For this review, take the finished solid that the model builds, in its own axes (mm). A direction names the side the tool comes from. Give positions to 0.01 mm unless a question says otherwise; leave off trailing zeros. Loops run counter-clockwise (first coordinate to the right, second up) from the corner with the lowest first, then second, coordinate; pieces in that order, holes last. Notation, with made-up numbers: (-32, -26.75) - (25, -26.75) arc R23 ccw to (25, 6.25) - close; hole circle Ø4 at (36.25, 19.5). An arc over 180 degrees is marked (long way). Use CSV: the item, a comma, the result in double quotes. Start each with the question number.
1. Wall thickness on line 1 (Y direction, x = 0.5, z = -2.25); line 2 (Z direction, x = 2.5, y = 14.5); line 3 (Y direction, x = 1, z = -1): over which ranges is each line inside the solid? List them lowest first.
2. Mouldability with a two-part tool opening along X and no side actions: class faces 1 (the cylindrical face through (0.41, 6.26, 1.86)), 2 (the flat face through (-1.25, 15.62, -2.33)), 3 (the flat face through (-2, 12.7, 1)) as pulls with the +X half, pulls with the -X half, needs draft (parallel to the pull), parting line crosses it, or undercut.
3. For pin 1 (2 mm diameter, centred on x = 1.5, z = 3, fed in from -Y); pin 2 (1 mm diameter, centred on x = 2.5, y = 9.5, fed in from -Z); pin 3 (2 mm diameter, centred on x = -4.5, y = 15, fed in from -Z); pin 4 (3 mm diameter, centred on y = 9.5, z = 0.5, fed in from -X) (3 decimals), all flat-tipped, find the tip position at first contact; note any pin that passes through.
4. Take a section at A-A on y = 4.75. Give the boundary of the cut face in (x, z) (3 decimals).
5. For faces 4 (the flat face through (0.74, 15.64, -2.29)), 5 (the flat face through (0, 0, 0)), list the 3-axis set-ups (+Z, -Z, +X, -X, +Y, -Y) from which the entire face can be reached by the end or side of a thin tool; tool diameter is ignored.
Autodesk Inventor part; units mm, degrees
ref_plane "YZ Plane" through (0, 0, 0) normal (1, 0, 0) x (0, 1, 0)
ref_plane "XZ Plane" through (0, 0, 0) normal (0, 1, 0) x (-1, 0, 0)
ref_plane "XY Plane" through (0, 0, 0) normal (0, 0, 1) x (1, 0, 0)
sketch "Sketch1" plane through (0, 0, 0) normal (0, 1, 0) x (-1, 0, 0)
  circle A0 centre (0, 0) radius 1.905
  dimension "d0" = 3.81
extrude "Extrusion1" add sketch "Sketch1" along normal blind 12.7
thread "Thread1"
sketch "Sketch2" plane through (0, 12.7, 0) normal (0, 1, 0) x (1, 0, 0)
  circle A0 centre (0, 0) radius 6.61892
extrude "Extrusion2" add sketch "Sketch2" along normal blind 5.08
fillet "Fillet1" radius 6.35 1 edges at (-6.6189, 17.78, 0)
sketch "Sketch3" plane through (0, 17.78, 0) normal (0, 1, 0) x (1, 0, 0)
  line L0 (-3.495957, -1.079634) -> (3.804424, -1.079634)
  line L1 (3.804424, -1.079634) -> (3.804424, 0.9254)
  line L2 (3.804424, 0.9254) -> (-3.495957, 0.9254)
  line L3 (-3.495957, 0.9254) -> (-3.495957, -1.079634)
  line L4 (-1.439512, -4.010068) -> (0.9254, -4.010068)
  line L5 (0.9254, -4.010068) -> (0.9254, 4.11289)
  line L6 (0.9254, 4.11289) -> (-1.439512, 4.11289)
  line L7 (-1.439512, 4.11289) -> (-1.439512, -4.010068)
  point P0 (0, 0)
sketch "Sketch3 outline for Extrusion3" plane through (0, 17.78, 0) normal (0, 1, 0) x (1, 0, 0)
  line L0 (-1.439512, 0.9254) -> (-3.495957, 0.9254)
  line L1 (-3.495957, 0.9254) -> (-3.495957, -1.079634)
  line L2 (-3.495957, -1.079634) -> (-1.439512, -1.079634)
  line L3 (-1.439512, -1.079634) -> (-1.439512, -4.010068)
  line L4 (-1.439512, -4.010068) -> (0.9254, -4.010068)
  line L5 (0.9254, -4.010068) -> (0.9254, -1.079634)
  line L6 (0.9254, -1.079634) -> (3.804424, -1.079634)
  line L7 (3.804424, -1.079634) -> (3.804424, 0.9254)
  line L8 (3.804424, 0.9254) -> (0.9254, 0.9254)
  line L9 (0.9254, 0.9254) -> (0.9254, 4.11289)
  line L10 (0.9254, 4.11289) -> (-1.439512, 4.11289)
  line L11 (-1.439512, 4.11289) -> (-1.439512, 0.9254)
extrude "Extrusion3" cut sketch "Sketch3 outline for Extrusion3" against normal blind 3.4925 draft -5
properties part number "tiny screw"
Check result:
1,line 1,"y = 12.7 to 14.29"
1,line 2,"z = -5.41 to -0.64, 0.79 to 5.41"
1,line 3,"y = 0 to 17.7"
2,face 1,"parting line crosses it"
2,face 2,"undercut"
2,face 3,"needs draft"
3,pin 1,"stops at y = 12.7"
3,pin 2,"passes through"
3,pin 3,"stops at z = -4.74"
3,pin 4,"stops at x = -1.905"
4,outline,"circle Ø3.81 at (0, 0)"
5,face 4,"+Y"
5,face 5,"+Z, -Z, +X, -X, -Y"
